The model under review builds one solid part; all positions refer to its coordinate system, in mm. A direction names the side the tool comes from. Coordinates: 2 decimals unless noted, no trailing zeros. Write each loop counter-clockwise with the first axis right and the second up, starting at its lowest first coordinate (ties: lowest second). Pieces come first, ordered by that corner, then holes. Notation, with made-up numbers: (29.25, 55) - (81.25, 55) arc R25 cw to (81.25, 81) - close; hole circle Ø8 at (55.5, -11.75). An arc over 180 degrees is marked (long way). Put each result on its own line as item: value. Start each with the question number.
Item 1: Consider section C-C on y = 0.15. State how many separate pieces and enclosed holes the cut face has, then the cut area to 3 significant figures.
Item 2: To check wall thickness, follow L1, parallel to X at y = 0.4, z = 12.15 (3 decimals); L2, parallel to X at y = -0.25, z = 0 (3 decimals); L3, parallel to Z at x = 23, y = 0.3. State the ranges of each line that lie inside material, in increasing order. Write a range as [from, to].
Item 3: Consider section A-A on z = 21.5. Give the boundary of the cut face in (x, y).
Item 4: For pin 1 (1.3 mm diameter, centred on x = -7, z = 0, fed in from +Y), flat-tipped, find the tip position at first contact; note if it passes through.
Item 5: Machinability: for faces 1 (the face through (-39, 0, -38)), 2 (the face through (20, 0, 13)), which of the approach directions +Z, -Z, +X, -X, +Y, -Y give a long, thin tool a straight path to every point of the face, cutting with its end or side? Answer none if there is none.
Item 6: Mouldability with a two-part tool opening along Z and no side actions: class faces 3 (the face through (-3.417, -0.011, -0.759)), 4 (the face through (-39, 0, 38)), 5 (the face through (-1, 0.75, -9)) as pulls with the +Z half, pulls with the -Z half, needs draft (parallel to the pull), parting line crosses it, or undercut.
Item 7: Consider section B-B on x = -20. Give the boundary of the cut face in (y, z), then the cut area to 3 significant figures.
```python
from build123d import *

# Parameters (mm, degrees)
SKETCH1_W               = 80
SKETCH1_H               = 80
BOSS_EXTRUDE1_DEPTH     = 0.75
FILLET1_R               = 5
FILLET3_R               = 5
FILLET4_R               = 5
FILLET5_R               = 5
CUT_EXTRUDE1_DEPTH      = 57.588426379
CUT_EXTRUDE1_DEPTH_BACK = 57.588426379
CUT_EXTRUDE2_DEPTH      = 57.588426379
CUT_EXTRUDE2_DEPTH_BACK = 57.588426379
SKETCH3_R               = 3.5
CUT_EXTRUDE3_DEPTH      = 57.588426379
CUT_EXTRUDE3_DEPTH_BACK = 57.588426379
SKETCH4_R               = 0.38
SKETCH4_R_2             = 0.65
SKETCH4_R_3             = 0.825


with BuildPart() as part:
    # Sketch1 → Boss-Extrude1 (new, symmetric)
    with BuildSketch(Plane(origin=(0, 0, 0), x_dir=(1, 0, 0), z_dir=(0, 1, 0))):
        Rectangle(SKETCH1_W, SKETCH1_H)
    extrude(amount=BOSS_EXTRUDE1_DEPTH, both=True)

    # Fillet1
    fillet1_edges = [part.edges().sort_by_distance(p)[0] for p in [
        (-40, 0, 40),
    ]]
    fillet(fillet1_edges, radius=FILLET1_R)

    # Fillet3
    fillet3_edges = [part.edges().sort_by_distance(p)[0] for p in [
        (-40, 0, -40),
    ]]
    fillet(fillet3_edges, radius=FILLET3_R)

    # Fillet4
    fillet4_edges = [part.edges().sort_by_distance(p)[0] for p in [
        (40, 0, -40),
    ]]
    fillet(fillet4_edges, radius=FILLET4_R)

    # Fillet5
    fillet5_edges = [part.edges().sort_by_distance(p)[0] for p in [
        (40, 0, 40),
    ]]
    fillet(fillet5_edges, radius=FILLET5_R)

    # Sketch2 → Cut-Extrude1 (cut, two sides: drawn at the far end of the back side and taken through both)
    with BuildSketch(Plane(origin=(0, 0.75, 0), x_dir=(1, 0, 0), z_dir=(0, 1, 0)).offset(-CUT_EXTRUDE1_DEPTH_BACK)):
        with BuildLine():
            Line((-24.5, 17.5), (-24.5, 22.5))
            ThreePointArc((-24.5, 22.5), (-20, 27), (-15.5, 22.5))
            Line((-15.5, 22.5), (-15.5, 17.5))
            ThreePointArc((-15.5, 17.5), (-20, 13), (-24.5, 17.5))
        make_face()
        with BuildLine():
            Line((-15.5, -17.5), (-15.5, -22.5))
            ThreePointArc((-15.5, -22.5), (-20, -27), (-24.5, -22.5))
            Line((-24.5, -22.5), (-24.5, -17.5))
            ThreePointArc((-24.5, -17.5), (-20, -13), (-15.5, -17.5))
        make_face()
        with BuildLine():
            Line((15.5, -17.5), (15.5, -22.5))
            ThreePointArc((15.5, -22.5), (20, -27), (24.5, -22.5))
            Line((24.5, -22.5), (24.5, -17.5))
            ThreePointArc((24.5, -17.5), (20, -13), (15.5, -17.5))
        make_face()
        with BuildLine():
            Line((24.5, 17.5), (24.5, 22.5))
            ThreePointArc((24.5, 22.5), (20, 27), (15.5, 22.5))
            Line((15.5, 22.5), (15.5, 17.5))
            ThreePointArc((15.5, 17.5), (20, 13), (24.5, 17.5))
        make_face()
    extrude(amount=CUT_EXTRUDE1_DEPTH + CUT_EXTRUDE1_DEPTH_BACK, mode=Mode.SUBTRACT)

    # Sketch3 → Cut-Extrude2 (cut, two sides: drawn at the far end of the back side and taken through both)
    with BuildSketch(Plane(origin=(0, 0.75, 0), x_dir=(1, 0, 0), z_dir=(0, 1, 0)).offset(-CUT_EXTRUDE2_DEPTH_BACK)):
        with Locations(Location((0, 0, 0), (0, 0, 270))):
            Circle(SKETCH3_R)
    extrude(amount=CUT_EXTRUDE2_DEPTH + CUT_EXTRUDE2_DEPTH_BACK, mode=Mode.SUBTRACT)

    # Sketch4 → Cut-Extrude3 (cut, two sides: drawn at the far end of the back side and taken through both)
    with BuildSketch(Plane(origin=(0, 0.75, 0), x_dir=(1, 0, 0), z_dir=(0, 1, 0)).offset(-CUT_EXTRUDE3_DEPTH_BACK)):
        with Locations(Location((-0.635, -12.15, 0), (0, 0, 270))):
            Circle(SKETCH4_R)
        with Locations(Location((-1.905, -12.15, 0), (0, 0, 270))):
            Circle(SKETCH4_R)
        with Locations(Location((-9.8, 0, 0), (0, 0, 270))):
            Circle(SKETCH4_R_2)
        with Locations(Location((-7, 0, 0), (0, 0, 270))):
            Circle(SKETCH4_R_3)
        with Locations(Location((7, 0, 0), (0, 0, 90))):
            Circle(SKETCH4_R_3)
        with Locations(Location((9.8, 0, 0), (0, 0, 90))):
            Circle(SKETCH4_R_2)
        with Locations(Location((0.635, -12.15, 0), (0, 0, 90))):
            Circle(SKETCH4_R)
        with Locations(Location((1.905, -12.15, 0), (0, 0, 90))):
            Circle(SKETCH4_R)
    extrude(amount=CUT_EXTRUDE3_DEPTH + CUT_EXTRUDE3_DEPTH_BACK, mode=Mode.SUBTRACT)


solid = part.part
```
Report:
1. separate pieces: 1
1. enclosed holes: 13
1. area: 5,900 mm²
2. L1: [-40, -2.285], [-1.525, -1.015], [-0.255, 0.255], [1.015, 1.525], [2.285, 40]
2. L2: [-40, -10.45], [-9.15, -7.825], [-6.175, -3.5], [3.5, 6.175], [7.825, 9.15], [10.45, 40]
2. L3: [-40, -25.85], [-14.15, 14.15], [25.85, 40]
3. outline: (-40, -0.75) - (-24.5, -0.75) - (-24.5, 0.75) - (-40, 0.75) - close; (-15.5, -0.75) - (15.5, -0.75) - (15.5, 0.75) - (-15.5, 0.75) - close; (24.5, -0.75) - (40, -0.75) - (40, 0.75) - (24.5, 0.75) - close
4. pin 1: through
5. face 1: -Z, -X, +Y, -Y
5. face 2: +Y, -Y
6. face 3: undercut
6. face 4: pulls with the +Z half
6. face 5: needs draft
7. outline: (-0.75, -40) - (0.75, -40) - (0.75, -27) - (-0.75, -27) - close; (-0.75, -13) - (0.75, -13) - (0.75, 13) - (-0.75, 13) - close; (-0.75, 27) - (0.75, 27) - (0.75, 40) - (-0.75, 40) - close
7. area: 78.0 mm²
